Can you work these out from the model? Positions are in its coordinate system, mm. Round coordinates to 2 decimals unless told otherwise and drop trailing zeros. Order: outer loops, then holes, each group sorted by start corner. A loop starts at its lowest first (then second) coordinate and runs counter-clockwise, first axis right, second up. Notation, with made-up numbers: (-5, 63) -> (51, 63) arc R34 ccw to (51, 99) -> close; hole circle Ø3 at (25, -10.75). An arc over 180 degrees is marked (long way). Use a Markdown table: item, result. Add a question column.
Q1. If we section it at A-A on z = 36: List the corners of the cut face in (x, y) for me.
Q2. I'm going to push a flat-ended pin straight in: pin 1 Ø18 at (x, y) = (1.5, -312.5) entering from +Z. Where does the tip first touch, or does it pass through?
Q3. I need wall thicknesses on line 1 along Y through (x, z) = (0, 37.75); line 2 along Y through (x, z) = (0, 7); line 3 along Z through (x, y) = (-4.5, -311). Which ranges of each line are inside material? Lowest first, please. Write a range as [from, to].
```python
from build123d import *

# Parameters (mm, degrees)
F0_W           = 76.2
F0_H           = 76.2
F1_DEPTH       = 762
F3_D           = 5.5
F3_CBORE_D     = 9.75
F3_CBORE_DEPTH = 5
F4_R           = 30.0187668276
F5_DEPTH       = 25.4
F6_T1_DEPTH    = 787.4
F6_T3_DEPTH    = 101.6


# Not quite as in the source:
# - a fillet or chamfer that OpenCascade refuses, or shapes differently, is made with other operations: its cross-section is extruded or revolved along the edge and cut away or added


with BuildPart() as f1:
    # F0 (on Front) → F1 (new body)
    with BuildSketch(Plane.XZ):
        with Locations((-2.2192886099, 13.3160627689)):
            Rectangle(F0_W, F0_H)
    extrude(amount=F1_DEPTH)

    # F3 (through all)
    with Locations(Plane.XY.offset(51.4160627689)):
        with Locations((0, -421.1068451405)):
            CounterBoreHole(F3_D / 2, F3_CBORE_D / 2, F3_CBORE_DEPTH)

    # F4 (on face) → F5 (cut)
    with BuildSketch(Plane.XY.offset(51.4160627689)):
        with Locations((0, -319.6821808815)):
            Circle(F4_R)
    extrude(amount=-F5_DEPTH, mode=Mode.SUBTRACT)

    # F6: fillet of radius 5.08 on 6 edges, made by hand

    # F6_s2 → F6_t1 (cut)
    with BuildSketch(Plane.XZ.offset(-12.7)):
        with BuildLine():
            ThreePointArc((30.8007113901, 51.4160627689), (34.3928138385, 49.9281652174), (35.8807113901, 46.3360627689))
            Line((35.8807113901, 46.3360627689), (35.8807113901, 51.4160627689))
            Line((35.8807113901, 51.4160627689), (30.8007113901, 51.4160627689))
        make_face()
        with BuildLine():
            ThreePointArc((-35.2392886099, 51.4160627689), (-38.8313910583, 49.9281652174), (-40.3192886099, 46.3360627689))
            Line((-40.3192886099, 46.3360627689), (-40.3192886099, 51.4160627689))
            Line((-40.3192886099, 51.4160627689), (-35.2392886099, 51.4160627689))
        make_face()
    extrude(amount=F6_T1_DEPTH, mode=Mode.SUBTRACT)

    # F6_s4 → F6_t3 (cut)
    with BuildSketch(Plane.YZ.offset(-53.0192886099)):
        with BuildLine():
            ThreePointArc((-5.08, 51.4160627689), (-1.4878975516, 49.9281652174), (0, 46.3360627689))
            Line((0, 46.3360627689), (0, 51.4160627689))
            Line((0, 51.4160627689), (-5.08, 51.4160627689))
        make_face()
        with BuildLine():
            ThreePointArc((-756.92, 51.4160627689), (-760.5121024484, 49.9281652174), (-762, 46.3360627689))
            Line((-762, 46.3360627689), (-762, 51.4160627689))
            Line((-762, 51.4160627689), (-756.92, 51.4160627689))
        make_face()
    extrude(amount=F6_T3_DEPTH, mode=Mode.SUBTRACT)


with BuildPart() as f6_tool6:
    # F6_s7 → F6_t8 (revolve)
    with BuildSketch(Plane.XZ.offset(421.1068451405)):
        with BuildLine():
            ThreePointArc((9.955, 51.4160627689), (6.3628975516, 49.9281652174), (4.875, 46.3360627689))
            Line((4.875, 46.3360627689), (4.875, 51.4160627689))
            Line((4.875, 51.4160627689), (9.955, 51.4160627689))
        make_face()
    revolve(axis=Axis((0, -421.1068451405, 51.4160627689), (0, 0, 1)))

    split(bisect_by=Plane.XY.offset(46.4160627689), keep=Keep.TOP)


with BuildPart() as f1_1:
    add(f1.part)

    # F6_t5: cut F6_tool6
    add(f6_tool6.part, mode=Mode.SUBTRACT)

    # F6_s10 → F6_t11 (revolve, cut)
    with BuildSketch(Plane.XZ.offset(319.6821808815)):
        with BuildLine():
            ThreePointArc((35.0987668276, 51.4160627689), (31.5066643792, 49.9281652174), (30.0187668276, 46.3360627689))
            Line((30.0187668276, 46.3360627689), (30.0187668276, 51.4160627689))
            Line((30.0187668276, 51.4160627689), (35.0987668276, 51.4160627689))
        make_face()
    revolve(axis=Axis((0, -319.6821808815, 51.4160627689), (0, 0, 1)), mode=Mode.SUBTRACT)


solid = f1_1.part
```
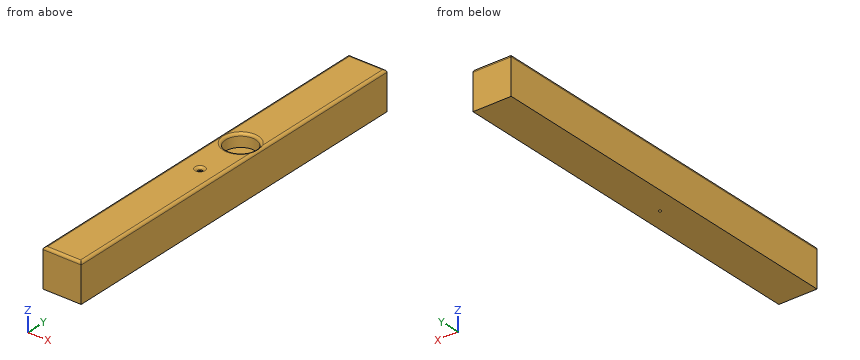
Answer below:
| question | item | result |
|---|---|---|
| 1 | outline | (-40.32, -762) -> (35.88, -762) -> (35.88, 0) -> (-40.32, 0) -> close; hole circle Ø60.04 at (0, -319.68); hole circle Ø5.5 at (0, -421.11) |
| 2 | pin 1 | z = 26.02 |
| 3 | line 1 | [-762, -423.86], [-418.36, -349.7], [-289.66, 0] |
| 3 | line 2 | [-762, -423.86], [-418.36, 0] |
| 3 | line 3 | [-24.78, 26.02] |
